Read the model definition and answer for the solid it produces. Units are mm, in the model's axes. A direction names the side the tool comes from. Coordinates: 2 decimals unless noted, no trailing zeros. Write each loop counter-clockwise with the first axis right and the second up, starting at its lowest first coordinate (ties: lowest second). Pieces come first, ordered by that corner, then holes.
from build123d import *

# Parameters (mm, degrees)
SKETCH1_W           = 45
SKETCH1_H           = 16
SKETCH1_R           = 3.5
SKETCH1_R_2         = 6
BOSS_EXTRUDE1_DEPTH = 3
SKETCH3_W           = 22
SKETCH3_H           = 3
BOSS_EXTRUDE3_DEPTH = 30


with BuildPart() as part:
    # Sketch1 → Boss-Extrude1 (new body)
    with BuildSketch(Plane.XY):
        with Locations((22.5, -8)):
            Rectangle(SKETCH1_W, SKETCH1_H)
        with Locations((5, -8)):
            Circle(SKETCH1_R, mode=Mode.SUBTRACT)
        with Locations((21, -8)):
            Circle(SKETCH1_R_2, mode=Mode.SUBTRACT)
        with Locations((37, -8)):
            Circle(SKETCH1_R_2, mode=Mode.SUBTRACT)
    extrude(amount=BOSS_EXTRUDE1_DEPTH)

    # Sketch3 → Boss-Extrude3 (add)
    with BuildSketch(Plane(origin=(0, 0, 0), x_dir=(-1, 0, 0), z_dir=(0, 0, -1))):
        with Locations((-4.75, -1.5)):
            Rectangle(SKETCH3_W, SKETCH3_H)
    extrude(amount=BOSS_EXTRUDE3_DEPTH)


solid = part.part
Item 1: For faces 5 (the flat face through (5, -3, -15)), 6 (the flat face through (15.75, -2, -15)), 7 (the flat face through (-3, -1, 0)), 8 (the flat face through (5, -1, -30)), 9 (the flat face through (17, -3, 3)), determine the directions among +Z, -Z, +X, -X, +Y, -Y from which every point of the face is accessible in a straight line to the end or side of a thin tool.
Item 2: Given pin 1 (8 mm diameter, centred on x = 30.5, y = -5.5, fed in from -Z); pin 2 (2.5 mm diameter, centred on y = -5.5, z = 1, fed in from -X); pin 3 (2.5 mm diameter, centred on y = -1.5, z = -15, fed in from +X), each flat-ended and moving along its own axis, determine where each tip first touches the part or whether it passes through.
Item 3: Determine the mould class of faces 1 (the flat face through (27.2, -7.9, 0)), 2 (the flat face through (-6.25, -2, -15)), 3 (the cylindrical face through (32.58, -3.94, 1.48)), 4 (the cylindrical face through (20.22, -2.05, 1.48)) for opening direction X: +X half, -X half, draft (parallel to the pull), parting line (faces both ways), or undercut.
Item 4: The part is cut by section D-D (z = -11.5). Give the vertices of the cut face in (x, y).
Item 5: The part is cut by section C-C (x = 37). Give the vertices of the cut face in (y, z), and give its area (3 significant figures).
Item 6: Find the intervals of material crossed by probe 1 along Y at (x, z) = (5, 1); probe 2 along Y at (x, z) = (37, 2.15); probe 3 along Z at (x, y) = (8, -10.25), in increasing order.
Item 7: The part is cut by section A-A (y = -8). Give the vertices of the cut face in (x, z), and give its area (3 significant figures).
Item 8: The part is cut by section B-B (x = 5). Give the vertices of the cut face in (y, z).
Answer:
1. face 5: -Z, +X, -X, -Y
1. face 6: -Z, +X, +Y, -Y
1. face 7: +Z, -X, +Y, -Y
1. face 8: -Z, +X, -X, +Y, -Y
1. face 9: +Z, +X, -X, +Y, -Y
2. pin 1: stops at z = 0
2. pin 2: stops at x = 0
2. pin 3: stops at x = 15.75
3. face 1: draft
3. face 2: -X half
3. face 3: undercut
3. face 4: undercut
4. outline: (-6.25, -3) - (15.75, -3) - (15.75, 0) - (-6.25, 0) - close
5. outline: (-16, 0) - (-14, 0) - (-14, 3) - (-16, 3) - close; (-2, 0) - (0, 0) - (0, 3) - (-2, 3) - close
5. area: 12.0 mm2
6. probe 1: y = -16 to -11.5, -4.5 to 0
6. probe 2: y = -16 to -14, -2 to 0
6. probe 3: z = 0 to 3
7. outline: (0, 0) - (1.5, 0) - (1.5, 3) - (0, 3) - close; (8.5, 0) - (15, 0) - (15, 3) - (8.5, 3) - close; (27, 0) - (31, 0) - (31, 3) - (27, 3) - close; (43, 0) - (45, 0) - (45, 3) - (43, 3) - close
7. area: 42.0 mm2
8. outline: (-16, 0) - (-11.5, 0) - (-11.5, 3) - (-16, 3) - close; (-4.5, 0) - (-3, 0) - (-3, -30) - (0, -30) - (0, 3) - (-4.5, 3) - close
